```python
from build123d import *

# Parameters (mm, degrees)
SKETCH1_W           = 45
SKETCH1_H           = 16
BOSS_EXTRUDE1_DEPTH = 14.1
FILLET1_R           = 8
SKETCH2_R           = 1.65
CUT_EXTRUDE1_DEPTH  = 21.1
SKETCH4_R           = 12.5
CUT_EXTRUDE2_DEPTH  = 2.65
BOSS_EXTRUDE3_DEPTH = 2.65
SKETCH7_R           = 0.5
CUT_EXTRUDE3_DEPTH  = 2.65
FILLET2_R           = 4
SKETCH8_R           = 2.55
CUT_EXTRUDE4_DEPTH  = 21.65
SKETCH9_R           = 2.85
CUT_EXTRUDE5_DEPTH  = 6


with BuildPart() as part:
    # Sketch1 → Boss-Extrude1 (new body)
    with BuildSketch(Plane.XY):
        with Locations((-14.5, 0)):
            Rectangle(SKETCH1_W, SKETCH1_H)
    extrude(amount=BOSS_EXTRUDE1_DEPTH)

    # Fillet1
    fillet1_edges = [part.edges().sort_by_distance(p)[0] for p in [
        (8, -8, 7.05),
        (8, 8, 7.05),
    ]]
    fillet(fillet1_edges, radius=FILLET1_R - 0.0001)  # a hair under: the kernel refuses the full size

    # Sketch2 → Cut-Extrude1 (cut)
    with BuildSketch(Plane.XZ.offset(8)):
        with Locations((-22.5, 7.05)):
            Circle(SKETCH2_R)
        with Locations((-31, 7.05)):
            Circle(SKETCH2_R)
    extrude(amount=-CUT_EXTRUDE1_DEPTH, mode=Mode.SUBTRACT)

    # Sketch4 → Cut-Extrude2 (cut)
    with BuildSketch(Plane(origin=(0, 0, 2.55), x_dir=(-1, 0, 0), z_dir=(0, 0, -1))):
        Circle(SKETCH4_R)
    cut_extrude2 = extrude(amount=-CUT_EXTRUDE2_DEPTH, mode=Mode.SUBTRACT)

    # Mirror1: Cut-Extrude2 across plane
    add(cut_extrude2.mirror(Plane(origin=(0, 0, 7.05), x_dir=(1, 0, 0), z_dir=(0, 0, -1))), mode=Mode.SUBTRACT)

    # Sketch6 → Boss-Extrude3 (add)
    with BuildSketch(Plane(origin=(0, 0, 0), x_dir=(-1, 0, 0), z_dir=(0, 0, -1))):
        with BuildLine():
            Line((0, 8), (12.68857754, 8))
            ThreePointArc((12.68857754, 8), (-15, 0), (12.68857754, -8))
            Line((12.68857754, -8), (0, -8))
            ThreePointArc((0, -8), (-5.656854249, -5.656854249), (-8, 0))
            ThreePointArc((-8, 0), (-5.656854249, 5.656854249), (0, 8))
        make_face()
    boss_extrude3 = extrude(amount=-BOSS_EXTRUDE3_DEPTH)

    # Sketch7 → Cut-Extrude3 (cut)
    with BuildSketch(Plane(origin=(0, 0, 0), x_dir=(-1, 0, 0), z_dir=(0, 0, -1))):
        with BuildLine():
            Line((-10.362969657, -6.989911293), (-13.099285488, -7.308126963))
            ThreePointArc((-13.099285488, -7.308126963), (-12.435563588, -8.387893552), (-11.68305604, -9.407773465))
            Line((-11.68305604, -9.407773465), (-10.362969657, -6.989911293))
        make_face()
        with BuildLine():
            Line((-8.991747504, -8.683229631), (-11.631234978, -9.471767147))
            ThreePointArc((-11.631234978, -9.471767147), (-10.790097005, -10.419875557), (-9.871921449, -11.293589638))
            Line((-9.871921449, -11.293589638), (-8.991747504, -8.683229631))
        make_face()
        with BuildLine():
            Line((-7.347315654, -10.11271243), (-9.809775279, -11.347612479))
            ThreePointArc((-9.809775279, -11.347612479), (-8.816778784, -12.135254916), (-7.76083352, -12.836255804))
            Line((-7.76083352, -12.836255804), (-7.347315654, -10.11271243))
        make_face()
        with BuildLine():
            Line((-5.479639335, -11.234925579), (-7.690250522, -12.878666348))
            ThreePointArc((-7.690250522, -12.878666348), (-6.575567202, -13.481910694), (-5.413936592, -13.988898834))
            Line((-5.413936592, -13.988898834), (-5.479639335, -11.234925579))
        make_face()
        with BuildLine():
            Line((-3.445466948, -12.015771199), (-5.337061395, -14.018408457))
            ThreePointArc((-5.337061395, -14.018408457), (-4.134560337, -14.418925439), (-2.90253994, -14.716496251))
            Line((-2.90253994, -14.716496251), (-3.445466948, -12.015771199))
        make_face()
        with BuildLine():
            ThreePointArc((-14.808828542, -2.387173479), (-14.554435894, -3.628828434), (-14.196129578, -4.844574801))
            Line((-14.196129578, -4.844574801), (-12.128696578, -3.024023695))
            Line((-12.128696578, -3.024023695), (-14.808828542, -2.387173479))
        make_face()
        with BuildLine():
            ThreePointArc((-14.998377485, 0.22061914), (-14.963460754, -1.046347106), (-14.821710057, -2.305842793))
            Line((-14.821710057, -2.305842793), (-12.469550628, -0.871955922))
            Line((-12.469550628, -0.871955922), (-14.998377485, 0.22061914))
        make_face()
        with Locations((-8.290375726, -5.591929035)):
            Circle(SKETCH7_R)
        with BuildLine():
            Line((-1.306605791, -12.431523692), (-2.821708358, -14.732208319))
            ThreePointArc((-2.821708358, -14.732208319), (-1.567926949, -14.917828431), (-0.302951081, -14.996940376))
            Line((-0.302951081, -14.996940376), (-1.306605791, -12.431523692))
        make_face()
        with BuildLine():
            ThreePointArc((-14.732208319, 2.821708358), (-14.917828431, 1.567926949), (-14.996940376, 0.302951081))
            Line((-14.996940376, 0.302951081), (-12.431523692, 1.306605791))
            Line((-12.431523692, 1.306605791), (-14.732208319, 2.821708358))
        make_face()
        Polygon((-11.419318221, -5.084208038), (-13.206757578, -7.320625266), (-14.277330492, -4.916079132), align=None)
    cut_extrude3 = extrude(amount=-CUT_EXTRUDE3_DEPTH, mode=Mode.SUBTRACT)

    # Mirror8: Boss-Extrude3, Cut-Extrude3 across plane
    add(boss_extrude3.mirror(Plane(origin=(0, 0, 7.05), x_dir=(1, 0, 0), z_dir=(0, 0, -1))))
    add(cut_extrude3.mirror(Plane(origin=(0, 0, 7.05), x_dir=(1, 0, 0), z_dir=(0, 0, -1))), mode=Mode.SUBTRACT)

    # Fillet2
    fillet2_edges = [part.edges().sort_by_distance(p)[0] for p in [
        (-37, 0, 14.1),
        (-37, 0, 0),
    ]]
    fillet(fillet2_edges, radius=FILLET2_R)

    # Sketch8 → Cut-Extrude4 (cut)
    with BuildSketch(Plane(origin=(0, 0, 0), x_dir=(-1, 0, 0), z_dir=(0, 0, -1))):
        Circle(SKETCH8_R)
    extrude(amount=-CUT_EXTRUDE4_DEPTH, mode=Mode.SUBTRACT)

    # Sketch9 → Cut-Extrude5 (cut)
    with BuildSketch(Plane(origin=(0, 8, 0), x_dir=(1, 0, 0), z_dir=(0, 1, 0))):
        with Locations(Location((-31, -7.05, 0), (0, 0, 270))):
            Circle(SKETCH9_R)
        with Locations(Location((-22.5, -7.05, 0), (0, 0, 270))):
            Circle(SKETCH9_R)
    extrude(amount=-CUT_EXTRUDE5_DEPTH, mode=Mode.SUBTRACT)


solid = part.part
```
Check sheet for the modelled part. Datum: model origin and axes. Units: mm. A direction names the side the tool comes from. Round coordinates to 2 decimals unless told otherwise and drop trailing zeros. Order: outer loops, then holes, each group sorted by start corner. A loop starts at its lowest first (then second) coordinate and runs counter-clockwise, first axis right, second up. Notation, with made-up numbers: (-32, 57) - (-26, 57) arc R26 cw to (-26, 73) - close; hole circle Ø1 at (-31.75, 3). An arc over 180 degrees is marked (long way). Write item = value, one per line.
Q1. Thickness scan on line 1 along Z through (x, y) = (-7, 3.5); line 2 along Z through (x, y) = (4, -9); line 3 along X through (y, z) = (4.1, 7.05). Record the ranges inside material, lowest first.
Computed:
line_1 = 0 to 2.55, 5.2 to 8.9, 11.55 to 14.1
line_2 = 0 to 2.65, 11.45 to 14.1
line_3 = -37 to -33.85, -28.15 to -25.35, -19.65 to 6.87
Q2. Section check D-D (x = -16). Record the boundary of the cut face in (y, z), and give its area (3 significant figures).
Computed:
outline = (-8, 0) - (8, 0) - (8, 14.1) - (-8, 14.1) - close
area = 226 mm^2
Q3. Section check A-A (z = 7.05). State how many separate pieces and enclosed holes the cut face has, and give its area (3 significant figures).
Computed:
separate_pieces = 3
enclosed_holes = 1
area = 538 mm^2
Q4. Go/stop test with flat-tipped pins: pin 1 (1.5 mm diameter, centred on y = -10, z = 8.5, fed in from -X); pin 2 (3 mm diameter, centred on x = -30, z = 6, fed in from +Y); pin 3 (2 mm diameter, centred on y = -10, z = 12, fed in from +X); pin 4 (6.5 mm diameter, centred on x = -31, z = 7.05, fed in from -Y). Record where each tip stops, or that it passes through.
Computed:
pin_1 = through
pin_2 = 8
pin_3 = 11.68
pin_4 = -8
Q5. Draft check along Z on faces 1 (the face through (10.29, -9.07, 1.31)), 2 (the face through (5.719, 5.594, 7.076)). Enter one of: pulls with the +Z half, pulls with the -Z half, needs draft (parallel to the pull), parting line crosses it, or undercut.
Computed:
face_1 = needs draft
face_2 = undercut
Q6. Tool access check on faces 3 (the face through (12.814, -5.002, 12.794)), 4 (the face through (4.378, -13.003, 1.306)), 5 (the face through (7.557, -11.494, 1.306)). Record the directions out of +Z, -Z, +X, -X, +Y, -Y that give a thin tool (end or side, any length) a straight path to the whole face; none if there is none.
Computed:
face_3 = +Z, -Z, +X
face_4 = +Z, -Z, -Y
face_5 = +Z, -Z
Q7. Section check C-C (x = -9). Record the boundary of the cut face in (y, z).
Computed:
outline = (-12, 0) - (12, 0) - (12, 2.65) - (8, 2.65) - (8, 2.55) - (-8, 2.55) - (-8, 2.65) - (-12, 2.65) - close; (-12, 11.45) - (-8, 11.45) - (-8, 11.55) - (8, 11.55) - (8, 11.45) - (12, 11.45) - (12, 14.1) - (-12, 14.1) - close; (-8, 5.2) - (8, 5.2) - (8, 8.9) - (-8, 8.9) - close
Q8. Section check B-B (x = -31). Record the boundary of the cut face in (y, z), and give its area (3 significant figures).
Computed:
outline = (-8, 0) - (8, 0) - (8, 4.2) - (2, 4.2) - (2, 5.4) - (-8, 5.4) - close; (-8, 8.7) - (2, 8.7) - (2, 9.9) - (8, 9.9) - (8, 14.1) - (-8, 14.1) - close
area = 158 mm^2
